```python
from build123d import *

# Parameters (mm, degrees)
F0_W = 80
F0_H = 80


# Not quite as in the source:
# - after a boolean that leaves OpenCascade's solid faulty, fix() repairs it


with BuildPart() as f1:
    # F0 (on Front) → F1 (revolve)
    with BuildSketch(Plane.XZ):
        with Locations((207.3035305738, 40)):
            Rectangle(F0_W, F0_H)
        Polygon((194.7596802331, -32.4445538099), (125.4776479304, -72.4445538099), (165.4776479304, -141.7265861126), (234.7596802331, -101.7265861126), align=None)
        with Locations((-40, -40)):
            Rectangle(F0_W, F0_H)
        Polygon((111.1079149462, -112.4445538099), (41.8258826435, -72.4445538099), (1.8258826435, -141.7265861126), (71.1079149462, -181.7265861126), align=None)
        Polygon((125.4776479304, 72.4445538099), (165.4776479304, 141.7265861126), (96.1956156276, 181.7265861126), (56.1956156276, 112.4445538099), align=None)
        Polygon((41.8258826435, 72.4445538099), (1.8258826435, 141.7265861126), (-67.4561496593, 101.7265861126), (-27.4561496593, 32.4445538099), align=None)
    revolve(axis=Axis((207.3035305738, 0, 0), (-1, 0, 0)))

    add(f1.part.fix(), mode=Mode.REPLACE)


solid = f1.part
```
Check sheet for the modelled part. Datum: model origin and axes. Units: mm. A direction names the side the tool comes from. Round coordinates to 2 decimals unless told otherwise and drop trailing zeros. Order: outer loops, then holes, each group sorted by start corner. A loop starts at its lowest first (then second) coordinate and runs counter-clockwise, first axis right, second up.
1) Go/stop test with flat-tipped pins: pin 1 Ø6 at (y, z) = (106.5, -120) entering from -X; pin 2 Ø5 at (x, y) = (17.5, 40) entering from +Z; pin 3 Ø6 at (y, z) = (-93.5, 18) entering from -X. Record where each tip stops, or that it passes through.
2) Tool access check on faces 1 (the cylindrical face through (-67.28, 78.1, 17.34)), 2 (the cylindrical face through (234.94, -78.1, -17.34)), 3 (the conical face through (83.04, -48.38, -153.62)). Record the directions out of +Z, -Z, +X, -X, +Y, -Y that give a thin tool (end or side, any length) a straight path to the whole face; none if there is none.
3) Section check A-A (x = -31.5). Record the boundary of the cut face in (y, z).
4) Scan lines: line 1 (X direction, y = -0.5, z = 21); line 2 (Y direction, x = 132, z = -39); line 3 (X direction, y = 25, z = 53.5). Record each from-to range of solid material in increasing order.
5) Section check B-B (x = 33). Record the boundary of the cut face in (y, z).
6) Mould release check, pull along X, two halves, no side actions. Record for faces 4 (the flat face through (0, -1, 1)), 5 (the flat face through (167.304, 1, 1)), 6 (the flat face through (247.304, 1, 1)), 7 (the flat face through (-80, -1, 1)): +X half, -X half, draft (parallel to the pull), parting line (faces both ways), or undercut.
Result:
1. pin 1: stops at x = 29.05
1. pin 2: stops at z = 147.01
1. pin 3: stops at x = -65.43
2. face 1: -X
2. face 2: +X
2. face 3: none
3. outline: circle Ø244.97 at (0, 0)
4. line 1: x = -80 to 0, 167.3 to 247.3
4. line 2: y = -156.26 to -56.53, 56.53 to 156.26
4. line 3: x = -80 to 18.63, 148.67 to 247.3
5. outline: circle Ø319.45 at (0, 0); hole circle Ø134.7 at (0, 0)
6. face 4: undercut
6. face 5: undercut
6. face 6: +X half
6. face 7: -X half
